Could you check a few things on this model? Use its own coordinates, in mm. A direction names the side the tool comes from. Give positions to 0.01 mm unless a question says otherwise; leave off trailing zeros. Loops run counter-clockwise (first coordinate to the right, second up) from the corner with the lowest first, then second, coordinate; pieces in that order, holes last. Notation, with made-up numbers: (88.25, 32.5) - (113.25, 32.5) arc R33 cw to (113.25, 71.5) - close; hole circle Ø9 at (-3, 2.25). An arc over 180 degrees is marked (long way). Write each question's results on one line, items separated by ' | '. Start each with the question number.
Autodesk Inventor part; units mm, degrees
ref_plane "Work Plane2" through (0, 18, 0) normal (0, 1, 0) x (1, 0, 0)
ref_plane "YZ Plane" through (0, 0, 0) normal (1, 0, 0) x (0, 1, 0)
ref_plane "XZ Plane" through (0, 0, 0) normal (0, 1, 0) x (-1, 0, 0)
sketch "Sketch1" plane through (0, 0, 0) normal (0, 1, 0) x (-1, 0, 0)
  line L0 (0, 0) -> (-95, 0)
  line L1 (-95, 0) -> (-95, -65)
  line L2 (-95, -65) -> (0, -65)
  line L3 (0, -65) -> (0, 0)
  line L4 (0, -65) -> (12.9904, -57.5)
  line L5 (12.9904, -57.5) -> (12.9904, -7.5)
  line L6 (12.9904, -7.5) -> (0, 0)
  line L7 (-95, -65) -> (-107.9904, -57.5)
  line L8 (-107.9904, -57.5) -> (-107.9904, -7.5)
  line L9 (-107.9904, -7.5) -> (-95, 0)
  dimension "d0" = 95
  dimension "d1" = 65
  dimension "d2" = 15
  dimension "d3" = 15
  dimension "d4" = 120
  dimension "d5" = 15
  dimension "d6" = 15
  dimension "d7" = 120
extrude "Extrusion1" add sketch "Sketch1" along normal blind 5
sketch "Sketch2" plane through (0, 5, 0) normal (0, 1, 0) x (1, 0, 0)
  line L0 (1.0001, 63.5) -> (94.0001, 63.5)
  line L1 (94.0001, 63.5) -> (94.0001, 1.5)
  line L2 (94.0001, 1.5) -> (1.0001, 1.5)
  line L3 (1.0001, 1.5) -> (1.0001, 63.5)
  line L4 (0, 0) -> (95, 0)
  line L5 (-12.9904, 57.5) -> (-12.9904, 7.5)
  dimension "d10" = 93
  dimension "d11" = 62
  dimension "d12" = 1.5
  dimension "d13" = 13.9905
extrude "Extrusion2" add sketch "Sketch2" along normal blind 8
sketch "Sketch4" plane through (0, 5, 0) normal (0, 1, 0) x (1, 0, 0)
  line L0 (-12.9904, 57.5) -> (-12.9904, 7.5)
  line L1 (-12.9904, 57.5) -> (-12.9904, 7.5)
  line L2 (-12.9904, 7.5) -> (0, 0)
  line L3 (0, 0) -> (95, 0)
  line L4 (95, 0) -> (107.9904, 7.5)
  line L5 (95, 0) -> (107.9904, 7.5)
  line L6 (107.9904, 7.5) -> (107.9904, 57.5)
  line L7 (107.9904, 57.5) -> (95, 65)
  line L8 (107.9904, 57.5) -> (95, 65)
  line L9 (95, 65) -> (0, 65)
  line L10 (95, 65) -> (0, 65)
  line L11 (0, 65) -> (-12.9904, 57.5)
  line L12 (-19.9904, 61.5415) -> (-19.9904, 3.4585)
  line L13 (114.9904, 61.5415) -> (114.9904, 3.4585)
  line L14 (-1.8756, 72) -> (96.8756, 72)
  line L15 (-19.9904, 61.5415) -> (-1.8756, 72)
  line L16 (96.8756, 72) -> (114.9904, 61.5415)
  line L17 (114.9904, 3.4585) -> (96.8756, -7)
  line L18 (-19.9904, 3.4585) -> (-1.8756, -7)
  line L19 (-1.8756, -7) -> (96.8756, -7)
  line L20 (95, 0) -> (107.9904, 7.5)
  line L21 (107.9904, 7.5) -> (107.9904, 57.5)
  line L22 (0, 0) -> (95, 0)
  dimension "d22" = 7
  dimension "d23" = 7
  dimension "d24" = 7
  dimension "d25" = 7
  dimension "d26" = 7
  dimension "d27" = 7
  dimension "d28" = 7
  dimension "d29" = 7
extrude "Extrusion4" add sketch "Sketch4" along normal blind 32 and the other way blind 5
sketch "Sketch5" plane through (0, 0, 0) normal (0, -1, 0) x (1, 0, 0)
  line L0 (2.4999, -63) -> (92.4999, -63)
  line L1 (92.4999, -63) -> (92.4999, -2)
  line L2 (92.4999, -2) -> (2.4999, -2)
  line L3 (2.4999, -2) -> (2.4999, -63)
  line L4 (0, 0) -> (95, 0)
  line L5 (-12.9904, -57.5) -> (-12.9904, -7.5)
  line L6 (96.8756, 7) -> (-1.8756, 7)
  line L7 (114.9904, -61.5415) -> (114.9904, -3.4585)
  line L8 (-1.8756, -72) -> (96.8756, -72)
  dimension "d34" = 61
  dimension "d35" = 90
  dimension "d44" = 22.4905
  dimension "d128" = 9
extrude "Extrusion5" cut sketch "Sketch5" against normal blind 11
chamfer "Chamfer1" distance 6 angle 45 8 edges at (47.5, 0, -72) (105.933, 0, -66.7707) (114.9904, 0, -32.5) (105.933, 0, 1.7707) (47.5, 0, 7) (-10.933, 0, 1.7707) (-19.9904, 0, -32.5) (-10.933, 0, -66.7707)
sketch "Sketch6" plane through (0, 0, 0) normal (0, -1, 0) x (1, 0, 0)
  line L0 (2.4999, -2) -> (-2.5001, -2)
  line L1 (-2.5001, -2) -> (-2.5001, -63.0139)
  line L2 (-2.5001, -63.0139) -> (2.4999, -63.0139)
  line L3 (2.4999, -63.0139) -> (2.4999, -2)
  line L4 (2.4999, -2) -> (92.4999, -2)
  line L5 (92.4999, -2) -> (97.4999, -2)
  line L6 (97.4999, -2) -> (97.4999, -63.0139)
  line L7 (97.4999, -63.0139) -> (92.4999, -63.0139)
  line L8 (92.4999, -63.0139) -> (92.4999, -2)
  point P0 (0, 0)
  dimension "d45" = 5
  dimension "d46" = 5
extrude "Extrusion6" cut sketch "Sketch6" against normal blind 2
sketch "Sketch7" plane through (0, 2, 0) normal (0, -1, 0) x (1, 0, 0)
  circle A0 centre (-0.0001, -6) radius 1.6
  circle A1 centre (94.9999, -6) radius 1.6
  circle A2 centre (-0.0001, -59.0139) radius 1.6
  circle A3 centre (94.9999, -59.0139) radius 1.6
  line L0 (94.0001, -63.5) -> (94.0001, -1.5)
  line L1 (2.4999, -2) -> (2.4999, -63)
  line L2 (97.4999, -2) -> (97.4999, -63.0139)
  line L3 (-2.5001, -2) -> (97.4999, -2)
  line L4 (-2.5001, -63.0139) -> (-2.5001, -2)
  line L5 (2.4999, -63.0139) -> (-2.5001, -63.0139)
  line L6 (92.4999, -63) -> (92.4999, -2)
  line L7 (97.4999, -63.0139) -> (92.4999, -63.0139)
  point P0 (0, 0)
  dimension "d49" = 3.2
  dimension "d50" = 2.5
  dimension "d51" = 2.5
  dimension "d52" = 4
  dimension "d53" = 0
  dimension "d54" = 2.5
  dimension "d55" = 4
  dimension "d56" = 2.5
  dimension "d57" = 4
extrude "Extrusion7" cut sketch "Sketch7" against normal blind 1 contours A0 | A1 L0 | L0 A1 | L0 A3 | A3 L0 | A2
sketch "Sketch8" plane through (0, 13, 0) normal (0, 1, 0) x (1, 0, 0)
  line L0 (5.0001, 60.5) -> (90.0001, 60.5)
  line L1 (90.0001, 60.5) -> (90.0001, 4.5)
  line L2 (90.0001, 4.5) -> (5.0001, 4.5)
  line L3 (5.0001, 4.5) -> (5.0001, 60.5)
  line L4 (96.8756, 72) -> (-1.8756, 72)
  line L5 (-19.9904, 61.5415) -> (-19.9904, 3.4585)
  circle A0 centre (28.5001, 57) radius 2.5
  circle A1 centre (28.5001, 8) radius 2.5
  circle A2 centre (86.5001, 57) radius 2.5
  circle A3 centre (86.5001, 8) radius 2.5
  circle A4 centre (28.5001, 8) radius 1.6
  circle A5 centre (86.5001, 8) radius 1.6
  circle A6 centre (86.5001, 57) radius 1.6
  circle A7 centre (28.5001, 57) radius 1.6
  circle A8 centre (28.5001, 57) radius 2.5
  point P0 (0, 0)
  dimension "d60" = 85
  dimension "d61" = 56
  dimension "d62" = 11.5
  dimension "d63" = 24.9905
  dimension "d65" = 3.5
  dimension "d66" = 5
  dimension "d68" = 3.5
  dimension "d69" = 3.5
  dimension "d70" = 3.5
  dimension "d71" = 58
  dimension "d72" = 58
  dimension "d75" = 3.5
  dimension "d76" = 3.5
  dimension "d100" = 3.2
  dimension "d101" = 3.2
  dimension "d102" = 3.2
  dimension "d103" = 3.2
extrude "Extrusion8" add sketch "Sketch8" along normal blind 5 contours A0 | A1 | A2 | A3 | A4 | A5 | A6 | A7
sketch "Sketch9" plane through (92.4999, 11, -63) normal (-1, 0, 0) x (0, 0, 1)
  circle A0 centre (49, -3) radius 1.5
  line L0 (61, 0) -> (0, 0)
  line L1 (61, -9) -> (61, 0)
  point P0 (63, -11)
  dimension "d77" = 3
  dimension "d78" = 3
  dimension "d79" = 12
extrude "Extrusion9" cut sketch "Sketch9" against normal blind 5
sketch "Sketch10" plane through (0, 37, 0) normal (0, 1, 0) x (1, 0, 0)
  line L0 (-12.9904, 7.5) -> (-12.9904, 57.5)
  line L1 (-12.9904, 7.5) -> (-16.4904, 1.4378)
  line L2 (-1.8756, -7) -> (-19.9904, 3.4585)
  line L3 (0, 0) -> (95, 0)
  line L4 (0, 0) -> (-3.486, -6.038)
  line L5 (-12.9904, 57.5) -> (0, 65)
  line L6 (-12.9904, 57.5) -> (-16.4904, 63.5622)
  line L7 (-1.8756, 72) -> (-19.9904, 61.5415)
  line L8 (0, 65) -> (-3.5, 71.0622)
  line L9 (0, 65) -> (95, 65)
  line L10 (95, 65) -> (98.5, 71.0622)
  line L11 (114.9904, 61.5415) -> (96.8756, 72)
  line L12 (107.9904, 57.5) -> (95, 65)
  line L13 (107.9904, 57.5) -> (111.4904, 63.5622)
  line L14 (95, 0) -> (107.9904, 7.5)
  line L15 (107.9904, 7.5) -> (111.4904, 1.4378)
  line L16 (95, 0) -> (98.5, -6.0622)
  line L17 (96.8756, -7) -> (114.9904, 3.4585)
  circle A0 centre (103.2452, 0.7189) radius 1.85
  circle A1 centre (103.2452, 64.2811) radius 1.6
  circle A2 centre (-8.2452, 64.2811) radius 1.65
  circle A3 centre (-8.2452, 0.7189) radius 1.75
  circle A4 centre (46.5, -3.5) radius 1.8
  circle A5 centre (46.5, 68.5) radius 1.7
  line L18 (0, 0) -> (-12.9904, 7.5)
  line L19 (-12.9904, 7.5) -> (0, 0)
  line L20 (0, 0) -> (0, -7)
  line L21 (-1.8756, -7) -> (96.8756, -7)
  line L22 (0, 65) -> (0, 72)
  dimension "d82" = 3.2
  dimension "d83" = 7.5
  dimension "d84" = 90
  dimension "d85" = 3.5
  dimension "d86" = 90
  dimension "d87" = 7.5
  dimension "d88" = 3.5
  dimension "d89" = 7.5
  dimension "d90" = 3.5
  dimension "d91" = 7.5
  dimension "d92" = 3.5
  dimension "d93" = 46.5
  dimension "d95" = 46.5
  dimension "d96" = 3.5
  dimension "d97" = 3.5
  dimension "d129" = 3.4
  dimension "d130" = 3.3
  dimension "d131" = 3.5
  dimension "d132" = 3.7
  dimension "d133" = 3.6
extrude "Extrusion10" cut sketch "Sketch10" against normal blind 3 contours A0 | A1 | A2 | A3 | A4 | A5
ref_plane "Work Plane2" through (0, 18, 0) normal (0, 1, 0) x (1, 0, 0)
sketch "Sketch14" plane through (0, 18, 0) normal (0, 1, 0) x (1, 0, 0)
  circle A0 centre (28.5001, 8) radius 1.6
  circle A1 centre (28.5001, 8) radius 2.5
  line L0 (28.5001, 8) -> (86.5001, 8)
  line L1 (86.5001, 8) -> (86.5001, 64)
  line L2 (86.5001, 64) -> (28.5001, 64)
  line L3 (28.5001, 64) -> (28.5001, 8)
  point P0 (0, 0)
  dimension "d108" = 3.2
  dimension "d109" = 0
  dimension "d110" = 0
  dimension "d117" = 56
  dimension "d118" = 58
extrude "Extrusion11" cut sketch "Sketch14" against normal blind 2.5 contours L0 L3 A0 | A0 L3 L0
sketch "Sketch15" plane through (86.5001, 18, -8) normal (0, 1, 0) x (1, 0, 0)
  circle A0 centre (0, 0) radius 1.6
  circle A1 centre (0, 49) radius 1.6
  circle A2 centre (0, 49) radius 2.5
  circle A3 centre (-58, 0) radius 1.6
  line L0 (-58, 0) -> (0, 0)
  line L1 (0, 0) -> (0, 49)
  line L2 (0, 49) -> (-58, 49)
  line L3 (-58, 49) -> (-58, 0)
  circle A4 centre (-58, 49) radius 1.6
  point P0 (-86.5001, -8)
  dimension "d113" = 3.2
  dimension "d114" = 3.2
  dimension "d115" = 5
  dimension "d116" = 0
  dimension "d119" = 49
  dimension "d120" = 58
  dimension "d121" = 3.2
extrude "Extrusion12" cut sketch "Sketch15" against normal blind 2.5 contours A0 L0 L1 | L1 L0 A0 | L1 L2 A1 | A1 L2 L1 | A4 L3 L2 | L2 L3 A4
sketch "Sketch16" plane through (107.9904, 5, -57.5) normal (-1, 0, 0) x (0, 0, 1)
  circle A0 centre (23.3152, 20.5) radius 7.8
  line L0 (0, 32) -> (50, 32)
  line L1 (0, 32) -> (50, 32)
  line L2 (57.5, 0) -> (50, 0)
  line L3 (50, 32) -> (50, 0)
  line L4 (50, 0) -> (0, 0)
  line L5 (0, 0) -> (0, 32)
  line L6 (0, 0) -> (0, 32)
  line L7 (-52.9421, -1.2141) -> (6.8536, -5)
  line L8 (6.8536, -5) -> (-57.6878, -5)
  line L9 (-57.6878, -5) -> (10.0174, -1.2141)
  point P0 (57.5, -5)
  dimension "d124" = 15.6
  dimension "d125" = 11.5
extrude "Extrusion13" cut sketch "Sketch16" against normal blind 10 contours A0
properties part number "FSCase_Bottom_v6"
Q1. I'm going to push flat-ended pins straight in: pin 1 Ø1 at (y, z) = (22, -62.5) entering from +X; pin 2 Ø4 at (x, z) = (21.5, -9) entering from -Y; pin 3 Ø5 at (x, z) = (86.5, -8) entering from +Y. Where does each tip first touch, or does it pass through?
Q2. Which directions (+Z, -Z, +X, -X, +Y, -Y) give clear straight access to the entire face, cutting with the end or side of a thin tool? Please do faces 1 (the face through (47, 5, -63)), 2 (the face through (104.33, 3.04, -64.28)), 3 (the face through (107.99, 17, -32)).
Q3. I want a section at A-A, the plane y = 8. List the corners of the cut face in (x, z) for me.
Q4. I want a section at D-D, the plane z = -34.5. List the corners of the cut face in (x, y) for me.
Q5. I need wall thicknesses on L1, parallel to X at y = 7, z = -15; L2, parallel to Z at x = 15, y = 6; L3, parallel to X at y = 6, z = -11. Which ranges of each line are inside material? Lowest first, please. Write a range as from..to.
Q6. If we mould it in two halves opening along X, with no side actions, what happens to faces 4 (the face through (105.81, 21.28, -66.84)), 5 (the face through (86, 15.5, -57)), 6 (the face through (-11.06, 21.283, -66.698))? For each: +X half, -X half, draft (parallel to the pull), parting line (faces both ways), or undercut.
Q7. I want a section at C-C, the plane z = -20. List the corners of the cut face in (x, y) for me.
Q8. I want a section at B-B, the plane x = 46.5. List the corners of the cut face in (y, z) for me, then the cut area to 3 significant figures.
Conclusion:
1) pin 1: x = 114.2 | pin 2: y = 11 | pin 3: y = 18
2) face 1: -Y | face 2: -Z, +X, -Y | face 3: +Y
3) outline: (-19.99, -61.54) - (-1.88, -72) - (96.88, -72) - (114.99, -61.54) - (114.99, -3.46) - (96.88, 7) - (-1.88, 7) - (-19.99, -3.46) - close; (1, -63.5) - (94, -63.5) - (94, -15.5) - (92.5, -15.5) - (92.5, -63) - (2.5, -63) - (2.5, -2) - (92.5, -2) - (92.5, -12.5) - (94, -12.5) - (94, -1.5) - (1, -1.5) - close; hole (-12.99, -57.5) - (0, -65) - (95, -65) - (107.99, -57.5) - (107.99, -7.5) - (95, 0) - (0, 0) - (-12.99, -7.5) - close
4) outline: (-19.99, 6) - (-13.99, 0) - (-2.5, 0) - (-2.5, 2) - (2.5, 2) - (2.5, 11) - (92.5, 11) - (92.5, 2) - (97.5, 2) - (97.5, 0) - (108.99, 0) - (114.99, 6) - (114.99, 17.71) - (107.99, 17.71) - (107.99, 5) - (94, 5) - (94, 13) - (1, 13) - (1, 5) - (-12.99, 5) - (-12.99, 37) - (-19.99, 37) - close; (107.99, 33.29) - (114.99, 33.29) - (114.99, 37) - (107.99, 37) - close
5) L1: -19.99..-12.99, 1..2.5, 107.99..114.99 | L2: -72..-65, -63.5..-63, -2..-1.5, 0..7 | L3: -19.99..-12.99, 1..2.5, 92.5..94, 107.99..114.99
6) face 4: +X half | face 5: undercut | face 6: -X half
7) outline: (-19.99, 6) - (-13.99, 0) - (-2.5, 0) - (-2.5, 2) - (2.5, 2) - (2.5, 11) - (92.5, 11) - (92.5, 2) - (97.5, 2) - (97.5, 0) - (108.99, 0) - (114.99, 6) - (114.99, 37) - (107.99, 37) - (107.99, 5) - (94, 5) - (94, 13) - (1, 13) - (1, 5) - (-12.99, 5) - (-12.99, 37) - (-19.99, 37) - close
8) outline: (0, -66) - (6, -72) - (37, -72) - (37, -70.2) - (34, -70.2) - (34, -66.8) - (37, -66.8) - (37, -65) - (5, -65) - (5, -63.5) - (13, -63.5) - (13, -1.5) - (5, -1.5) - (5, 0) - (37, 0) - (37, 1.7) - (34, 1.7) - (34, 5.3) - (37, 5.3) - (37, 7) - (6, 7) - (0, 1) - (0, -2) - (11, -2) - (11, -63) - (0, -63) - close | area: 611 mm^2
